Design review of the part built by this model. Coordinates are the model's own, in mm. Face numbers are marked on the shaded views. A direction names the side the tool comes from. Coordinates: 2 decimals unless noted, no trailing zeros. Order: outer loops, then holes, each group sorted by start corner. A loop starts at its lowest first (then second) coordinate and runs counter-clockwise, first axis right, second up. Notation, with made-up numbers: M 16.5,74 L 50.5,74 A24 ccw 50.5,95 Z; hole C 88.25,76.25 d4. An arc over 180 degrees is marked long. Answer as a JSON object with one key per item and string values.
from build123d import *

# Parameters (mm, degrees)
SKETCH001_W   = 40
SKETCH001_H   = 50
SKETCH001_R   = 2.25
SKETCH001_R_2 = 2.5
PAD001_DEPTH  = 3
SKETCH_R      = 2.5
PAD_DEPTH     = 5
PAD002_DEPTH  = 5
SKETCH003_R   = 1.4
SKETCH003_R_2 = 2.7
POCKET_DEPTH  = 8.001
FILLET_R      = 1
FILLET001_R   = 1
FILLET002_R   = 1
FILLET003_R   = 1
FILLET004_R   = 10


with BuildPart() as part:
    # Sketch001 → Pad001 (new body)
    with BuildSketch(Plane.XY):
        with Locations((0, 5)):
            Rectangle(SKETCH001_W, SKETCH001_H)
        Circle(SKETCH001_R, mode=Mode.SUBTRACT)
        with Locations((0, 25)):
            Circle(SKETCH001_R_2, mode=Mode.SUBTRACT)
        with Locations((0, -15)):
            Circle(SKETCH001_R_2, mode=Mode.SUBTRACT)
    extrude(amount=-PAD001_DEPTH)

    # Sketch → Pad (join)
    with BuildSketch(Plane.XY):
        with BuildLine():
            ThreePointArc((-10.337741, -1.838777), (-0.081993, -10.49968), (10.307764, -2))
            Line((7.228416, -2), (10.307764, -2))
            Line((7.228416, -2), (7.228416, 2))
            Line((10.307764, 2), (7.228416, 2))
            ThreePointArc((10.307764, 2), (-0.081993, 10.49968), (-10.337741, 1.838777))
            Line((-10.337741, 1.838777), (-7.2711, 1.838777))
            Line((-7.2711, -1.838777), (-7.2711, 1.838777))
            Line((-7.2711, -1.838777), (-10.337741, -1.838777))
        make_face()
        Circle(SKETCH_R, mode=Mode.SUBTRACT)
    extrude(amount=PAD_DEPTH)

    # Sketch002 → Pad002 (join)
    with BuildSketch(Plane.XY):
        with BuildLine():
            ThreePointArc((-4.812647, -13.8), (0, -20.155888), (4.812647, -13.8))
            Line((4.812647, -13.8), (-4.812647, -13.8))
        make_face()
        with BuildLine():
            ThreePointArc((4.853864, 13.8), (0, 20), (-4.853864, 13.8))
            Line((4.853864, 13.8), (-4.853864, 13.8))
        make_face()
    extrude(amount=PAD002_DEPTH)

    # Sketch003 (on Face23 of Pad002) → Pocket (cut, through all)
    with BuildSketch(Plane.XY.offset(5)):
        with Locations((0, 16.5)):
            Circle(SKETCH003_R)
        with Locations((0, -15)):
            Circle(SKETCH003_R_2)
    extrude(amount=-POCKET_DEPTH, mode=Mode.SUBTRACT)

    # Fillet
    fillet_edges = [part.edges().sort_by_distance(p)[0] for p in [
        (-0.081993, -10.49968, 5),
        (-0.081993, 10.49968, 5),
    ]]
    fillet(fillet_edges, radius=FILLET_R)

    # Fillet001
    fillet001_edges = [part.edges().sort_by_distance(p)[0] for p in [
        (8.257752, 2, 5),
        (7.228416, 0, 5),
        (8.257752, -2, 5),
    ]]
    fillet(fillet001_edges, radius=FILLET001_R)

    # Fillet002
    fillet002_edges = [part.edges().sort_by_distance(p)[0] for p in [
        (-8.295724, 1.838777, 5),
    ]]
    fillet(fillet002_edges, radius=FILLET002_R)

    # Fillet003
    fillet003_edges = [part.edges().sort_by_distance(p)[0] for p in [
        (-7.2711, 0, 5),
        (-8.295724, -1.838777, 5),
    ]]
    fillet(fillet003_edges, radius=FILLET003_R)

    # Fillet004
    fillet004_edges = [part.edges().sort_by_distance(p)[0] for p in [
        (20, -20, -1.5),
        (-20, -20, -1.5),
        (20, 30, -1.5),
        (-20, 30, -1.5),
    ]]
    fillet(fillet004_edges, radius=FILLET004_R)


solid = part.part
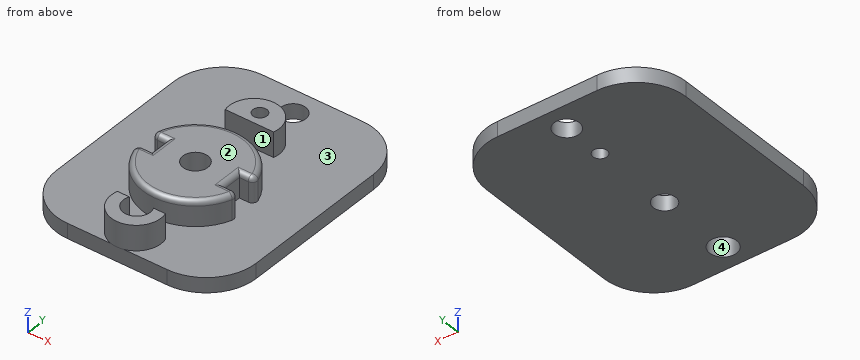
1) Add section C-C (z = -1.5). State the section outline as (x, y) points.
Taken from the geometry:
{"outline": "M -20,-10 A10 ccw -10,-20 L 10,-20 A10 ccw 20,-10 L 20,20 A10 ccw 10,30 L -10,30 A10 ccw -20,20 Z; hole C 0,-15 d5.4; hole C 0,25 d5; hole C 0,0 d4.5; hole C 0,16.5 d2.8"}
2) Tool access review of the marked faces 3 and 4: name each direction out of +Z, -Z, +X, -X, +Y, -Y from which nothing blocks a thin tool from reaching the whole face with its end or side.
Taken from the geometry:
{"face 3": "+Z", "face 4": "+Z, -Z"}
3) Insertion check: pin 1 Ø3 at (x, y) = (0, -15) entering from -Z; pin 2 Ø4 at (y, z) = (-1, 3) entering from +X; pin 3 Ø2 at (y, z) = (4, 4) entering from -X; pin 4 Ø4 at (y, z) = (0, 2.5) entering from -X. Each pin has a flat end and moves straight along its axis. Give the tip position at first contact, or say it passes through.
Taken from the geometry:
{"pin 1": "passes through", "pin 2": "stops at x = 10.01", "pin 3": "stops at x = -10.05", "pin 4": "stops at x = -9.61"}
4) Mouldability with a two-part tool opening along Y and no side actions: class the marked faces 1 and 2 as released by +Y, released by -Y, zero draft, split by the parting line, or undercut.
Taken from the geometry:
{"face 1": "undercut", "face 2": "zero draft"}
5) Add section D-D (x = 0). Count the separate pieces of the cut face and the enclosed holes in it, and give its area (3 significant figures).
Taken from the geometry:
{"separate pieces": "5", "enclosed holes": "0", "area": "206 mm2"}
6) Add section A-A (z = 3). State the section outline as (x, y) points.
Taken from the geometry:
{"outline": "M -10.02,-3.14 A10.5 ccw 9.96,-3.32 A1 ccw 9.01,-2 L 7.23,-2 L 7.23,2 L 9.01,2 A1 ccw 9.96,3.32 A10.5 ccw -10.02,3.14 A1 ccw -9.07,1.84 L -7.27,1.84 L -7.27,-1.84 L -9.07,-1.84 A1 ccw Z; M -4.85,13.8 L 4.85,13.8 A5 ccw long Z; M -4.81,-13.8 A5 ccw long 4.81,-13.8 L 2.42,-13.8 A2.7 cw long -2.42,-13.8 Z; hole C 0,0 d5; hole C 0,16.5 d2.8"}
7) Add section B-B (y = -17). State the section outline as (x, z) points, and give its area (3 significant figures).
Taken from the geometry:
{"outline": "M -17.14,-3 L -1.81,-3 L -1.81,5 L -4.65,5 L -4.65,0 L -17.14,0 Z; M 1.81,-3 L 17.14,-3 L 17.14,0 L 4.65,0 L 4.65,5 L 1.81,5 Z", "area": "120 mm2"}
8) To check wall thickness, follow L1, parallel to Y at x = 0, z = -0.9; L2, parallel to Y at x = 0, z = 2.6; L3, parallel to X at y = -15, z = 0.75. State the ranges of each line that lie inside material, in increasing order.
Taken from the geometry:
{"L1": "y = -20 to -17.7, -12.3 to -2.25, 2.25 to 15.1, 17.9 to 22.5, 27.5 to 30", "L2": "y = -20.16 to -17.7, -10.5 to -2.5, 2.5 to 10.5, 13.8 to 15.1, 17.9 to 20", "L3": "x = -5 to -2.7, 2.7 to 5"}
